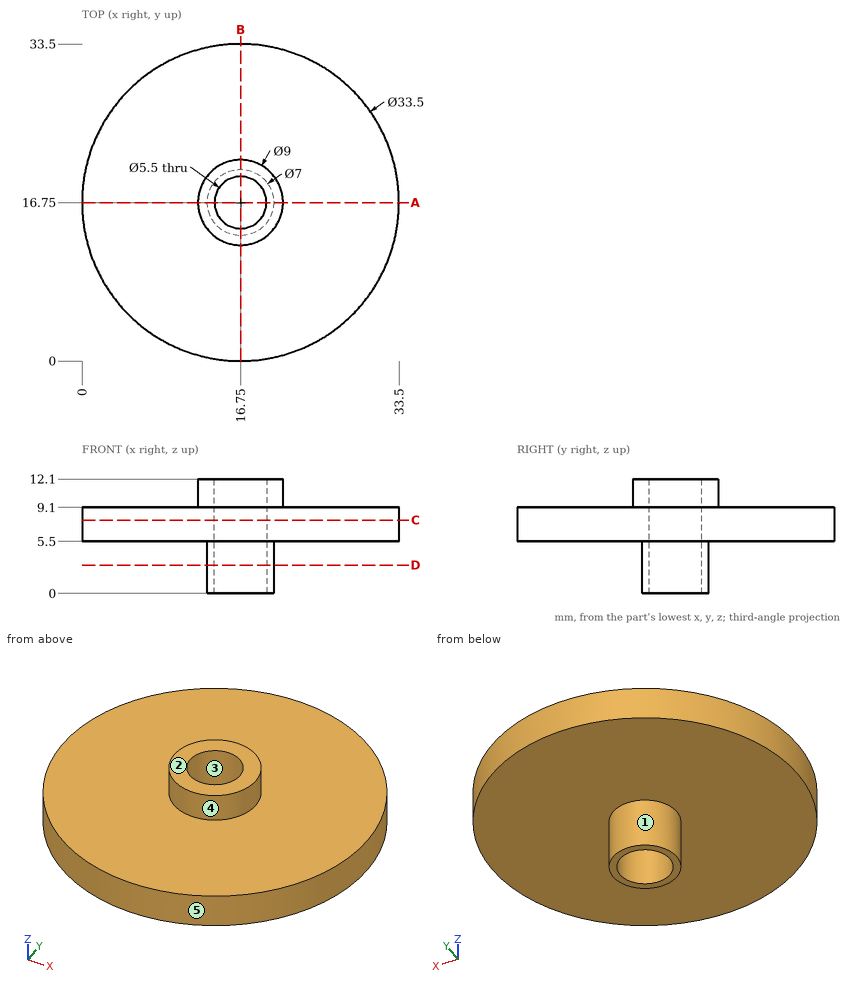
The drawing under review shows one solid part. Ordinate dimensions are in mm from its lowest x, y, z. A direction names the side the tool comes from. Give positions to 0.01 mm unless a question says otherwise; leave off trailing zeros. Loops run counter-clockwise (first coordinate to the right, second up) from the corner with the lowest first, then second, coordinate; pieces in that order, holes last. Notation, with made-up numbers: M -6.5,11.25 L 25.5,11.25 A18 cw 25.5,18.25 Z; hole C 68,64.25 d1. An arc over 180 degrees is marked long. One line per question, with ' | ' between items. Start each with the question number.
1. Add section A-A (y = 16.75). Write out the cut boundary in (x, z).
2. To check wall thickness, follow L1, parallel to Y at x = 16.75, z = 2.5; L2, parallel to Z at x = 7, y = 15.5; L3, parallel to Z at x = 20.5, y = 18. State the ranges of each line that lie inside material, in increasing order.
3. For the marked faces 4 and 5, list the 3-axis set-ups (+Z, -Z, +X, -X, +Y, -Y) from which the entire face can be reached by the end or side of a thin tool; tool diameter is ignored.
4. Add section C-C (z = 7.75). Write out the cut boundary in (x, y).
5. Insertion check: P1, Ø1.5, axis at x = 6.5, z = 6, coming from the -Y side; P2, Ø4, axis at x = 23, z = 5, coming from the +Y side; P3, Ø3, axis at x = 23, z = 4.5, coming from the +Y side. Each pin has a flat end and moves straight along its axis. Give the tip position at first contact, or say it passes through.
6. The part is to be moulded in two halves that separate along Y. For the marked faces 1, 2 and 3, say which applies: released by +Y, released by -Y, zero draft, split by the parting line, or undercut.
7. Add section D-D (z = 3). Write out the cut boundary in (x, y), plus the area to 3 significant figures.
Worked out:
1) outline: M 0,5.5 L 13.25,5.5 L 13.25,0 L 14,0 L 14,12.1 L 12.25,12.1 L 12.25,9.1 L 0,9.1 Z; M 19.5,0 L 20.25,0 L 20.25,5.5 L 33.5,5.5 L 33.5,9.1 L 21.25,9.1 L 21.25,12.1 L 19.5,12.1 Z
2) L1: y = 13.25 to 14, 19.5 to 20.25 | L2: z = 5.5 to 9.1 | L3: z = 5.5 to 12.1
3) face 4: +Z | face 5: +Z, -Z
4) outline: C 16.75,16.75 d33.5; hole C 16.75,16.75 d5.5
5) P1: stops at y = 2.95 | P2: stops at y = 32.94 | P3: stops at y = 32.69
6) face 1: split by the parting line | face 2: zero draft | face 3: undercut
7) outline: C 16.75,16.75 d7; hole C 16.75,16.75 d5.5 | area: 14.7 mm²
